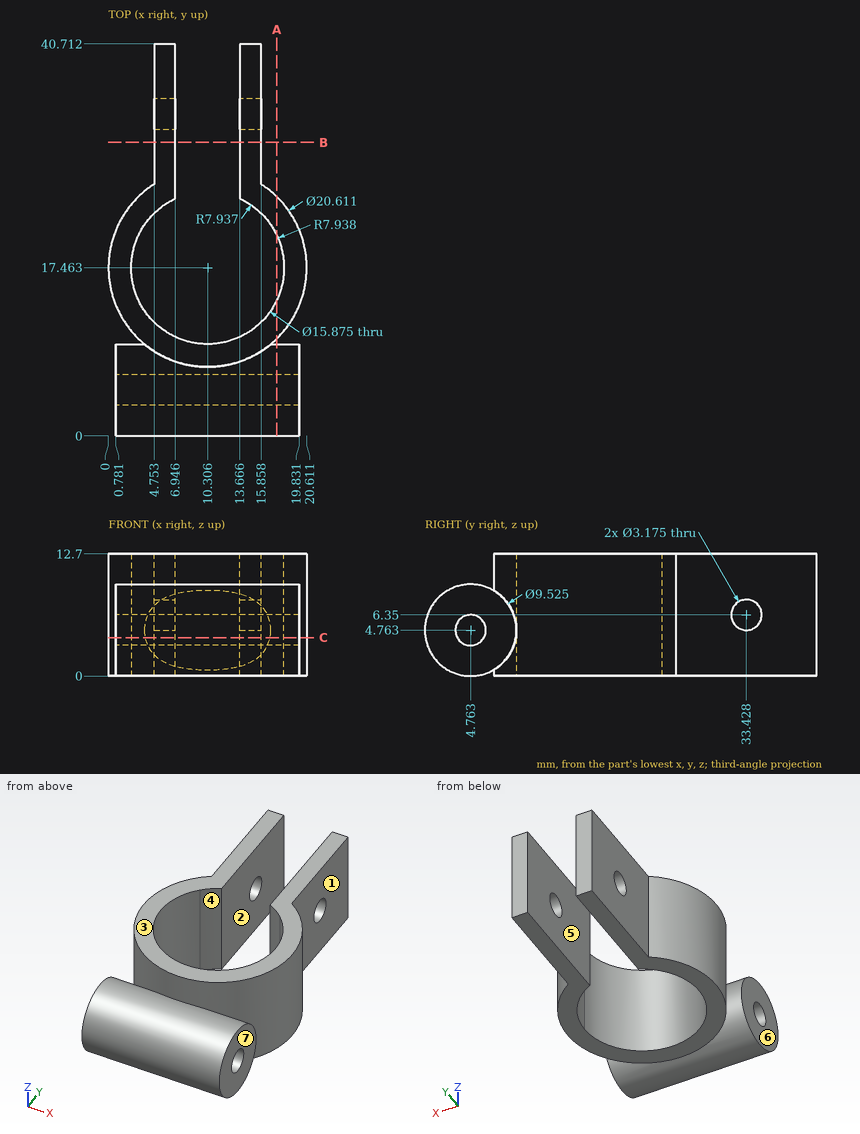
Geometry: see drawing. Coordinates: mm, zero at the bounding-box minimum. A direction names the side the tool comes from. Give positions to 0.01 mm unless a question says otherwise; leave off trailing zeros. Order: outer loops, then holes, each group sorted by start corner. A loop starts at its lowest first (then second) coordinate and runs counter-clockwise, first axis right, second up. Notation, with made-up numbers: (-34.5, 31.5) -> (17.5, 31.5) arc R12 cw to (17.5, 46.5) -> close; hole circle Ø8 at (-4, 66.25). An arc over 180 degrees is marked (long way). Write item = value, one per line.
Q1. Cut plane A-A, the plane x = 17.5. State how many separate pieces and enclosed holes the cut face has.
Data:
separate_pieces = 3
enclosed_holes = 1
Q2. Cut plane B-B, the plane y = 30.5. Output: boundary loops of the cut face in (x, z) (1 decimal).
Data:
outline = (4.8, 0) -> (6.9, 0) -> (6.9, 12.7) -> (4.8, 12.7) -> close; (13.7, 0) -> (15.9, 0) -> (15.9, 12.7) -> (13.7, 12.7) -> close
Q3. Cut plane C-C, the plane z = 4. Output: boundary loops of the cut face in (x, y) (1 decimal).
Data:
outline = (0.8, 0.1) -> (19.8, 0.1) -> (19.8, 3.4) -> (0.8, 3.4) -> close; (0.8, 6.2) -> (19.8, 6.2) -> (19.8, 9.5) -> (16.8, 9.5) arc R10.3 ccw to (15.9, 26.1) -> (15.9, 40.7) -> (13.7, 40.7) -> (13.7, 24.7) arc R7.9 cw to (15.9, 23.1) arc R7.9 cw to (18.2, 17.5) arc R7.9 cw (long way) to (4.8, 23.1) arc R7.9 cw to (6.9, 24.7) -> (6.9, 40.7) -> (4.8, 40.7) -> (4.8, 26.1) arc R10.3 ccw to (3.8, 9.5) -> (0.8, 9.5) -> close
Q4. Set-up query: the marked faces 4, 5, 6 and 7. Return all of +Z, -Z, +X, -X, +Y, -Y with unobstructed straight access to the full face (end or side cutting, diameter ignored); none if empty.
Data:
face_4 = +Z, -Z
face_5 = +Z, -Z, +Y
face_6 = +Z, -Z, -X, -Y
face_7 = +Z, -Z, +X, -Y
Q5. Pull-direction query (X, two-part tool) for the marked faces 1, 2 and 3; classes: released by +X, released by -X, zero draft, split by the parting line, or undercut.
Data:
face_1 = released by +X
face_2 = undercut
face_3 = zero draft
Q6. Material intervals for line 1 (Y direction, x = 6, z = 4) (1 decimal); line 2 (X direction, y = 28, z = 3.75) (1 decimal); line 3 (X direction, y = 5, z = 9), sorted ascending. Write a range as from..to.
Data:
line_1 = 0.1..3.4, 6.2..10.8, 24.1..40.7
line_2 = 4.8..6.9, 13.7..15.9
line_3 = 0.78..19.83
Q7. Pin query (flat end, axial travel): pin 1 (4 mm diameter, centred on y = 30, z = 7.5, fed in from -X); pin 2 (4 mm diameter, centred on y = 31.5, z = 7.5, fed in from +X); pin 3 (7.5 mm diameter, centred on y = 4, z = 5.5, fed in from +X). Return the tip coordinate at first contact, or that it passes through.
Data:
pin_1 = 4.75
pin_2 = 15.86
pin_3 = 19.83
